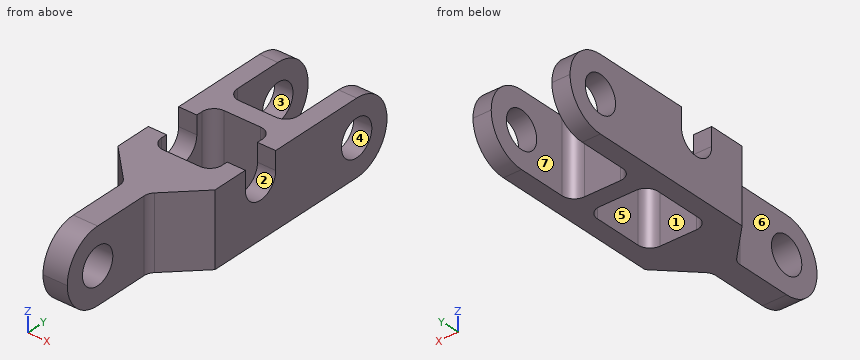
from build123d import *

# Parameters (mm, degrees)
F1_DEPTH = 9.525
F2_R     = 1.5875
F3_R     = 4.76249
F4_R     = 2.38125
F5_DEPTH = 12.7


# Not quite as in the source:
# - a fillet or chamfer is up to 0.001 mm smaller than in the source, because OpenCascade refuses the exact size


with BuildPart() as f1:
    # F0 (on Top) → F1 (new body)
    with BuildSketch(Plane.XY):
        Polygon((0, 12.7), (0, 0), (3.175, 0), (3.175, 12.7), (7.9375, 17.4625), (7.9375, 44.45), (5.55625, 44.45), (5.55625, 31.75), (1.5875, 31.75), (-2.38125, 31.75), (-2.38125, 44.45), (-4.7625, 44.45), (-4.7625, 17.4625), align=None)
        Polygon((-2.38125, 29.36875), (1.5875, 29.36875), (5.55625, 29.36875), (5.55625, 19.84375), (-2.38125, 19.84375), align=None, mode=Mode.SUBTRACT)
    extrude(amount=F1_DEPTH)

    # F2
    f2_edges = [f1.edges().sort_by_distance(p)[0] for p in [
        (-2.38125, 31.75, 4.7625),
        (5.55625, 31.75, 4.7625),
        (5.55625, 29.36875, 4.7625),
        (-2.38125, 29.36875, 4.7625),
        (-2.38125, 19.84375, 4.7625),
        (5.55625, 19.84375, 4.7625),
        (0, 12.7, 4.7625),
        (3.175, 12.7, 4.7625),
    ]]
    fillet(f2_edges, radius=F2_R)

    # F3 (radius 4.7625 in the source; OpenCascade refuses exactly that, so slightly less here)
    f3_edges = [f1.edges().sort_by_distance(p)[0] for p in [
        (1.5875, 0, 9.525),
        (1.5875, 0, 0),
        (-3.571875, 44.45, 9.525),
        (-3.571875, 44.45, 0),
        (6.746875, 44.45, 9.525),
        (6.746875, 44.45, 0),
    ]]
    fillet(f3_edges, radius=F3_R)

    # F4 (on face) → F5 (cut, through all)
    with BuildSketch(Plane(origin=(-4.7625, 0, 0), x_dir=(0, -1, 0), z_dir=(-1, 0, 0))):
        with Locations((-39.6875, 4.7625)):
            Circle(F4_R)
        with Locations((-4.7625, 4.7625)):
            Circle(F4_R)
        with BuildLine():
            Line((-22.225, 9.525), (-26.9875, 9.525))
            Line((-26.9875, 9.525), (-26.9875, 7.14375))
            ThreePointArc((-26.9875, 7.14375), (-24.60625, 4.7625), (-22.225, 7.14375))
            Line((-22.225, 7.14375), (-22.225, 9.525))
        make_face()
    extrude(amount=-F5_DEPTH, mode=Mode.SUBTRACT)


solid = f1.part
Part model, mm, in its own coordinate system. Face numbers are marked on the shaded views. A direction names the side the tool comes from. Give positions to 0.01 mm unless a question says otherwise; leave off trailing zeros. Loops run counter-clockwise (first coordinate to the right, second up) from the corner with the lowest first, then second, coordinate; pieces in that order, holes last. Notation, with made-up numbers: (57.25, 76) -> (63.25, 76) arc R5 ccw to (63.25, 84) -> close; hole circle Ø8 at (-28.5, 44). An arc over 180 degrees is marked (long way). Write each question's results on one line, items separated by ' | '. Start each with the question number.
Q1. Band-saw the part on A-A on x = 1. Count the separate pieces of the cut face and the enclosed holes in it, plus the area to 3 significant figures.
Q2. Which spindle directions (+Z, -Z, +X, -X, +Y, -Y) get a long thin tool onto all of the face, cutting with end or side? Do the marked faces 5, 6 and 7. Say none if no direction does.
Q3. Band-saw the part on B-B on y = 42.5. List the corners of the cut face in (x, z).
Q4. Pin check, flat tips, straight feed: P1, Ø3, axis at y = 3.5, z = 3, coming from the -X side; P2, Ø1.9, axis at x = -3, z = 8.5, coming from the -Y side; P3, Ø4, axis at x = 0.5, z = 6, coming from the +Y side; P4, Ø3, axis at y = 39.69, z = 4.76, coming from the -X side. Stop position of each tip, or through.
Q5. Band-saw the part on C-C on x = -1.5. List the corners of the cut face in (y, z) (1 decimal), plus the area to 3 significant figures.
Q6. Wall check: L1, parallel to Y at x = 1.75, z = 4.75; L2, parallel to X at y = 27, z = 4.75; L3, parallel to Y at x = 2.5, z = 3.5. Give the ranges that are in metal, low to high.
Q7. Pull direction Z, two halves, no side cores. Call the marked faces 1, 2, 3 and 4: +Z half, -Z half, draft (parallel to the pull), parting line (faces both ways), or undercut.
Results are:
1) separate pieces: 2 | enclosed holes: 1 | area: 184 mm²
2) face 5: +Z, -Z | face 6: +Z, -Z, -X, -Y | face 7: +Z, -Z, +Y
3) outline: (-4.76, 0.92) -> (-2.38, 0.92) -> (-2.38, 8.61) -> (-4.76, 8.61) -> close; (5.56, 0.92) -> (7.94, 0.92) -> (7.94, 8.61) -> (5.56, 8.61) -> close
4) P1: stops at x = 0 | P2: stops at y = 14.75 | P3: stops at y = 31.92 | P4: passes through
5) outline: (14.2, 0) -> (20, 0) -> (20, 9.5) -> (14.2, 9.5) -> close; (29.2, 0) -> (31.9, 0) -> (31.9, 9.5) -> (29.2, 9.5) -> close | area: 81.2 mm²
6) L1: y = 0 to 2.38, 7.14 to 19.84, 29.37 to 31.75 | L2: x = -4.76 to -2.38, 5.56 to 7.94 | L3: y = 0.17 to 2.74, 6.78 to 19.84, 29.37 to 31.75
7) face 1: draft | face 2: +Z half | face 3: undercut | face 4: undercut
